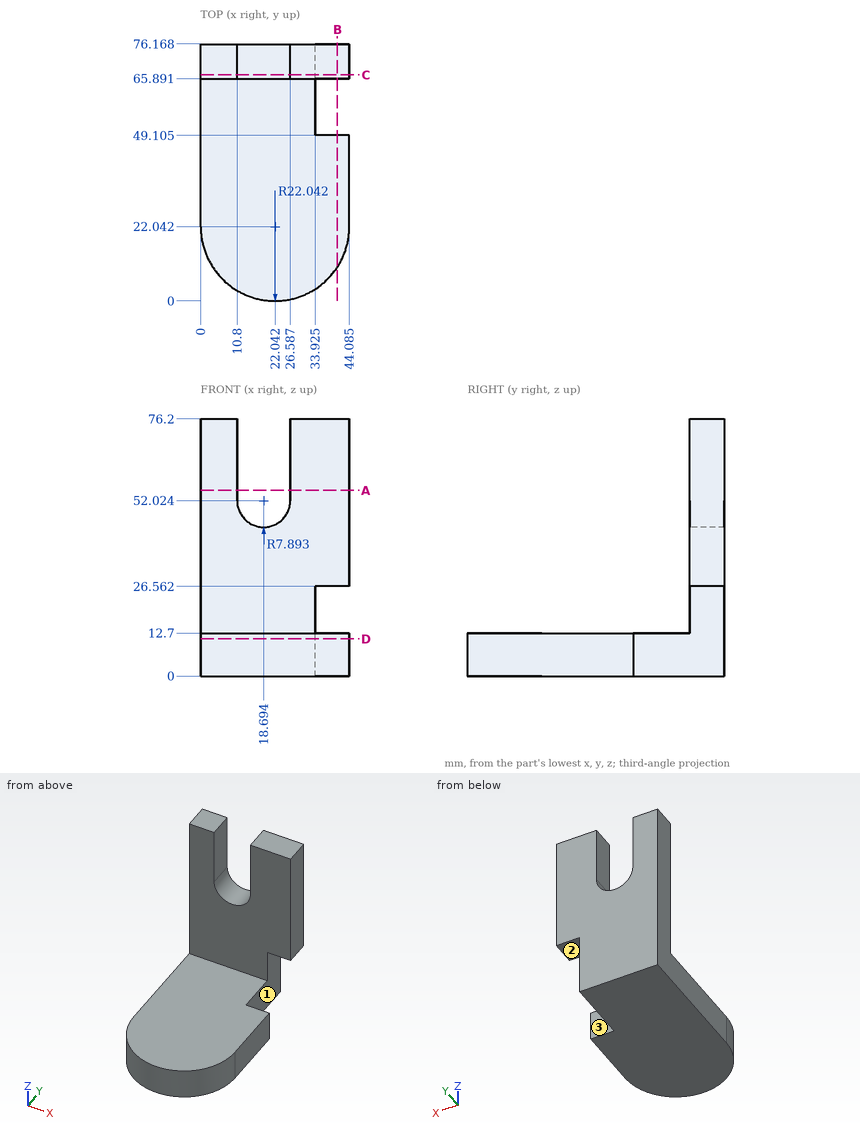
The figure shows three views and two pictorial views of one solid part (mm, origin at its lowest corner). Answer the questions. A direction names the side the tool comes from. Give positions to 0.01 mm unless a question says otherwise; leave off trailing zeros. Write each loop counter-clockwise with the first axis right and the second up, starting at its lowest first coordinate (ties: lowest second). Pieces come first, ordered by that corner, then holes. Notation, with made-up numbers: (84.5, 85) - (142.5, 85) arc R12 cw to (142.5, 95) - close; hole circle Ø6 at (85.25, -11). An arc over 180 degrees is marked (long way). Use one line per item in the form item = value. Start each with the question number.
1) Find section A-A on z = 55. Determine the outline of the cut face in (x, y) (1 decimal).
2) Find section C-C on y = 67. Determine the outline of the cut face in (x, z) (1 decimal), plus the area to 3 significant figures.
3) Consider line 1 along X through (y, z) = (73.5, 61.5) (1 decimal); line 2 along Y through (x, z) = (6.5, 73); line 3 along Z through (x, y) = (20.5, 34). Determine where each line is inside the solid, lowest interval first. Write a range as from..to.
4) Find section B-B on x = 40.5. Determine the outline of the cut face in (y, z) (1 decimal).
5) Flat-ended cylindrical pins translate along their axes: pin 1 Ø8 at (x, z) = (22, 13) entering from -Y; pin 2 Ø1.5 at (x, z) = (36.5, 24.5) entering from +Y; pin 3 Ø10 at (x, y) = (36, 18) entering from +Z; pin 4 Ø5 at (x, y) = (38.5, 71.5) entering from -Z. Find the tip coordinate at first contact, or state that the pin passes through.
6) Find section D-D on z = 11. Determine the outline of the cut face in (x, y) (1 decimal), plus the area to 3 significant figures.
7) A tool of negligible diameter and unlimited length cuts with its end or side. For the marked faces 1, 2 and 3, from which of +Z, -Z, +X, -X, +Y, -Y can it reach the whole face along a straight path? Write none if from no direction.
Geometry results:
q1.outline = (0, 65.9) - (10.8, 65.9) - (10.8, 76.2) - (0, 76.2) - close; (26.6, 65.9) - (44.1, 65.9) - (44.1, 76.2) - (26.6, 76.2) - close
q2.outline = (0, 0) - (33.9, 0) - (33.9, 26.6) - (44.1, 26.6) - (44.1, 76.2) - (26.6, 76.2) - (26.6, 52) arc R7.9 cw to (10.8, 52) - (10.8, 76.2) - (0, 76.2) - close
q2.area = 2,610 mm2
q3.line_1 = 0..10.8, 26.6..44.1
q3.line_2 = 65.89..76.17
q3.line_3 = 0..12.7
q4.outline = (10, 0) - (49.1, 0) - (49.1, 12.7) - (10, 12.7) - close; (65.9, 26.6) - (76.2, 26.6) - (76.2, 76.2) - (65.9, 76.2) - close
q5.pin_1 = 0
q5.pin_2 = through
q5.pin_3 = 12.7
q5.pin_4 = 26.56
q6.outline = (0, 22) arc R22 ccw to (44.1, 22) - (44.1, 49.1) - (33.9, 49.1) - (33.9, 76.2) - (0, 76.2) - close
q6.area = 2,870 mm2
q7.face_1 = -Z, +X, +Y
q7.face_2 = -Z, +X, +Y, -Y
q7.face_3 = +Z, -Z, +X, +Y
